from build123d import *

# Parameters (mm, degrees)
SKETCH1_W           = 230
SKETCH1_H           = 90
BOSS_EXTRUDE1_DEPTH = 5
FILLET1_R           = 20
CUT_EXTRUDE1_REACH  = 125.592
SKETCH2_R           = 11


with BuildPart() as part:
    # Sketch1 → Boss-Extrude1 (new body)
    with BuildSketch(Plane.XY):
        Rectangle(SKETCH1_W, SKETCH1_H)
    extrude(amount=BOSS_EXTRUDE1_DEPTH)

    # Fillet1
    fillet1_edges = [part.edges().sort_by_distance(p)[0] for p in [
        (-115, 45, 2.5),
        (115, 45, 2.5),
    ]]
    fillet(fillet1_edges, radius=FILLET1_R)

    # Sketch2 → Cut-Extrude1 (cut, up to next)
    with BuildSketch(Plane.XY.offset(5), mode=Mode.PRIVATE) as cut_extrude1_sk1:
        with Locations((-20.95, 10)):
            Circle(SKETCH2_R)
    cut_extrude1_tool1 = extrude(cut_extrude1_sk1.sketch, amount=-CUT_EXTRUDE1_REACH, mode=Mode.PRIVATE) & part.part
    # Sketch2 → Cut-Extrude1 (cut, up to next)
    with BuildSketch(Plane.XY.offset(5), mode=Mode.PRIVATE) as cut_extrude1_sk2:
        with Locations((20.95, 10)):
            Circle(SKETCH2_R)
    cut_extrude1_tool2 = extrude(cut_extrude1_sk2.sketch, amount=-CUT_EXTRUDE1_REACH, mode=Mode.PRIVATE) & part.part
    add(cut_extrude1_tool1.solids().sort_by_distance((-20.95, 10, 5))[0], mode=Mode.SUBTRACT)
    add(cut_extrude1_tool2.solids().sort_by_distance((20.95, 10, 5))[0], mode=Mode.SUBTRACT)


solid = part.part
Verification items for the finished model (mm, model axes). Give positions to 0.01 mm unless a question says otherwise; leave off trailing zeros. Order: outer loops, then holes, each group sorted by start corner. A loop starts at its lowest first (then second) coordinate and runs counter-clockwise, first axis right, second up. Notation, with made-up numbers: (8.25, 21) -> (56.25, 21) arc R10 ccw to (56.25, 38) -> close; hole circle Ø7 at (78.5, 14). An arc over 180 degrees is marked (long way). Answer as CSV lines item,"result".
Q1. Scan lines: probe 1 along Y at (x, z) = (20.95, 3.3); probe 2 along X at (y, z) = (7, 3.45); probe 3 along X at (y, z) = (16, 1). Record each from-to range of solid material in increasing order.
Solutions:
probe 1,"y = -45 to -1, 21 to 45"
probe 2,"x = -115 to -31.53, -10.37 to 10.37, 31.53 to 115"
probe 3,"x = -115 to -30.17, -11.73 to 11.73, 30.17 to 115"
Q2. Sectioned sample at C-C on y = 10. Record the cut outline in (x, z).
Solutions:
outline,"(-115, 0) -> (-31.95, 0) -> (-31.95, 5) -> (-115, 5) -> close; (-9.95, 0) -> (9.95, 0) -> (9.95, 5) -> (-9.95, 5) -> close; (31.95, 0) -> (115, 0) -> (115, 5) -> (31.95, 5) -> close"
Q3. Sectioned sample at B-B on z = 1.35. Record the cut outline in (x, y).
Solutions:
outline,"(-115, -45) -> (115, -45) -> (115, 25) arc R20 ccw to (95, 45) -> (-95, 45) arc R20 ccw to (-115, 25) -> close; hole circle Ø22 at (-20.95, 10); hole circle Ø22 at (20.95, 10)"
Q4. Sectioned sample at D-D on y = 34.5. Record the cut outline in (x, z), plus the area to 3 significant figures.
Solutions:
outline,"(-112.6, 0) -> (112.6, 0) -> (112.6, 5) -> (-112.6, 5) -> close"
area,"1,130 mm²"
Q5. Release check for a two-part mould opening along X. For faces 1 (the flat face through (115, -10, 2)), 2 (the cylindrical face through (-23.33, -0.74, 2.54)), 3 (the flat face through (-2, 1, 0)) record: +X half, -X half, draft (parallel to the pull), parting line (faces both ways), or undercut.
Solutions:
face 1,"+X half"
face 2,"undercut"
face 3,"draft"
Q6. Depth check by flat-ended pin: pin 1 (13 mm diameter, centred on x = 20.95, y = 10, fed in from -Z). Enter the tip coordinate at first touch or a pass-through.
Solutions:
pin 1,"passes through"
Q7. Sectioned sample at A-A on x = -20.95. Record the cut outline in (y, z).
Solutions:
outline,"(-45, 0) -> (-1, 0) -> (-1, 5) -> (-45, 5) -> close; (21, 0) -> (45, 0) -> (45, 5) -> (21, 5) -> close"
